from build123d import *

# Parameters (mm, degrees)
ESBO_O1_R                = 3.45
RESSALTO_EXTRUS_O1_DEPTH = 1.4
ESBO_O2_R                = 3.45
RESSALTO_EXTRUS_O2_DEPTH = 2.4
FURO1_D                  = 4.95
FURO1_DEPTH              = 2
FURO2_D                  = 4.6
FURO2_DEPTH              = 1
FURO3_D                  = 2.1
BOSS_EXTRUDE1_DEPTH      = 2
SKETCH3_R                = 3
BOSS_EXTRUDE2_DEPTH      = 16
SKETCH4_RX               = 2.25
SKETCH4_RY               = 1.25
BOSS_EXTRUDE3_DEPTH      = 7
FILLET3_SIZE             = 2.5


with BuildPart() as part:
    # Esboço1 → Ressalto-extrusão1 (new body)
    with BuildSketch(Plane(origin=(0, 0, 0), x_dir=(1, 0, 0), z_dir=(0, 1, 0))):
        with Locations(Location((0, 0, 0), (0, 0, 270))):
            Circle(ESBO_O1_R)
    extrude(amount=-RESSALTO_EXTRUS_O1_DEPTH)

    # Esboço2 → Ressalto-extrusão2 (add)
    with BuildSketch(Plane.XZ.offset(1.4)):
        with Locations(Location((0, 0, 0), (0, 0, 90))):
            Circle(ESBO_O2_R)
    extrude(amount=RESSALTO_EXTRUS_O2_DEPTH)

    # Furo1
    with Locations(Plane(origin=(0, -3.8, 0), x_dir=(-1, 0, 0), z_dir=(0, -1, 0))):
        with Locations((0, 0)):
            Hole(FURO1_D / 2, depth=FURO1_DEPTH)

    # Furo2
    with Locations(Plane(origin=(0, 0, 0), x_dir=(1, 0, 0), z_dir=(0, 1, 0))):
        with Locations((0, 0)):
            Hole(FURO2_D / 2, depth=FURO2_DEPTH)

    # Furo3 (through all)
    with Locations(Plane(origin=(0, 0, 0), x_dir=(1, 0, 0), z_dir=(0, 1, 0))):
        with Locations((0, 0)):
            Hole(FURO3_D / 2)

    # Sketch2 → Boss-Extrude1 (add)
    with BuildSketch(Plane(origin=(0, 0, 0), x_dir=(1, 0, 0), z_dir=(0, 1, 0))):
        with BuildLine():
            Line((20.067369497, 2.999243463), (0.154910769, 3.446520369))
            ThreePointArc((0.154910769, 3.446520369), (2.493686243, 2.384120157), (3.45, 0))
            ThreePointArc((3.45, 0), (2.493686243, -2.384120157), (0.154910769, -3.446520369))
            Line((0.154910769, -3.446520369), (20.067369497, -2.999243463))
            ThreePointArc((20.067369497, -2.999243463), (23, 0), (20.067369497, 2.999243463))
        make_face()
    extrude(amount=-BOSS_EXTRUDE1_DEPTH)

    # Sketch3 → Boss-Extrude2 (add)
    with BuildSketch(Plane.XZ.offset(2)):
        with Locations(Location((20.067369497, 0, 0), (0, 0, 270))):
            Circle(SKETCH3_R)
    extrude(amount=-BOSS_EXTRUDE2_DEPTH)

    # Sketch4 → Boss-Extrude3 (add)
    with BuildSketch(Plane.XZ.offset(2)):
        with Locations((12.067369497, 0)):
            Ellipse(SKETCH4_RX, SKETCH4_RY)
    extrude(amount=BOSS_EXTRUDE3_DEPTH)

    # Fillet3
    # a fillet whose section is not a circle: 2.5 mm, written as the material it takes off along each edge
    with BuildSketch(Plane(origin=(20.067369497, 14, 0), x_dir=(0, 0, -1), z_dir=(-1, 0, 0))) as fillet3_piece_1:
        with BuildLine():
            Bezier((3, FILLET3_SIZE), (3, 0), (3 - FILLET3_SIZE, 0), weights=[1, 0.176470588, 1])
            Line((3 - FILLET3_SIZE, 0), (3, 0))
            Line((3, 0), (3, FILLET3_SIZE))
        make_face()
    revolve(axis=Axis((20.067369497, 14, 0), (0, -1, 0)), mode=Mode.SUBTRACT)


solid = part.part
Geometry: final body of the model. Coordinates: model frame, mm. A direction names the side the tool comes from. Coordinates: 2 decimals unless noted, no trailing zeros. Write each loop counter-clockwise with the first axis right and the second up, starting at its lowest first coordinate (ties: lowest second). Pieces come first, ordered by that corner, then holes. Notation, with made-up numbers: (27, -8) - (55, -8) arc R23 cw to (55, 12) - close; hole circle Ø9 at (51, 29.25). An arc over 180 degrees is marked (long way). Return JSON: item names as keys, results as strings.
Item 1: Reachability of faces 1 (the face through (2.3, -3.8, 1.5)), 2 (the face through (1, -1.8, 1)), 3 (the face through (-1, -1, -1)) from +Z, -Z, +X, -X, +Y, -Y: full face, straight path, thin tool, end or side. Return the list, or none.
Completed:
{"face 1": "+Z, -Z, -X, -Y", "face 2": "-Y", "face 3": "+Y"}
Item 2: Section query C-C (x = 4). Output: boundary loops of the cut face in (y, z).
Completed:
{"outline": "(-2, -3.36) - (0, -3.36) - (0, 3.36) - (-2, 3.36) - close"}
Item 3: Pin query (flat end, axial travel): pin 1 Ø1.5 at (x, z) = (5, 1) entering from +Y; pin 2 Ø2.5 at (x, z) = (0, 0) entering from +Y; pin 3 Ø1 at (x, y) = (16.5, 5) entering from -Z; pin 4 Ø4 at (x, z) = (1, -0.5) entering from -Y. Return the tip coordinate at first contact, or that it passes through.
Completed:
{"pin 1": "stops at y = 0", "pin 2": "stops at y = -1", "pin 3": "passes through", "pin 4": "stops at y = -3.8"}
Item 4: Section query A-A (x = 8.5). Output: boundary loops of the cut face in (y, z).
Completed:
{"outline": "(-2, -3.26) - (0, -3.26) - (0, 3.26) - (-2, 3.26) - close"}
Item 5: Section query B-B (y = 8). Output: boundary loops of the cut face in (x, z), and give its area (3 significant figures).
Completed:
{"outline": "circle Ø6 at (20.07, 0)", "area": "28.3 mm2"}
Item 6: Pull-direction query (Z, two-part tool) for faces 4 (the face through (-3.42, -2.3, -0.45)), 5 (the face through (1.825, -0.507, 1.4)), 6 (the face through (20, 14, 0)); classes: +Z half, -Z half, draft (parallel to the pull), parting line (faces both ways), or undercut.
Completed:
{"face 4": "parting line", "face 5": "undercut", "face 6": "draft"}
Item 7: Line query: L1, parallel to Z at x = 0, y = -0.5; L2, parallel to Z at x = 0, y = -1.35; L3, parallel to Y at x = 0.25, z = -2.5. Output: solid intervals per line, ascending.
Completed:
{"L1": "z = -3.45 to -2.3, 2.3 to 3.45", "L2": "z = -3.45 to -1.05, 1.05 to 3.45", "L3": "y = -3.8 to 0"}
